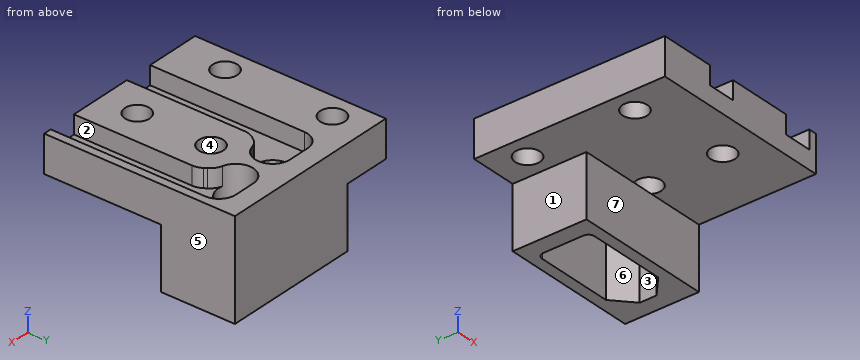
Autodesk Inventor part; units mm, degrees
ref_plane "YZ Plane" through (0, 0, 0) normal (1, 0, 0) x (0, 1, 0)
ref_plane "XZ Plane" through (0, 0, 0) normal (0, 1, 0) x (-1, 0, 0)
ref_plane "XY Plane" through (0, 0, 0) normal (0, 0, 1) x (1, 0, 0)
sketch "Эскиз1" plane through (0, 0, 0) normal (0, 0, 1) x (1, 0, 0)
  line L0 (-10, -10.5115) -> (10, -10.5115)
  line L1 (10, -10.5115) -> (10, 10.5115)
  line L2 (10, 10.5115) -> (-10, 10.5115)
  line L3 (-10, 10.5115) -> (-10, -10.5115)
  line L4 (-10, -10.5115) -> (10, 10.5115) construction
  line L5 (10, -10.5115) -> (-10, 10.5115) construction
  point P0 (0, 0)
  dimension "d0" = 20
  dimension "d1" = 21.023
extrude "Выдавливание1" add sketch "Эскиз1" along normal blind 6
sketch "Эскиз2" plane through (0, 0, 6) normal (0, 0, 1) x (1, 0, 0)
  circle A0 centre (2.5, 4.5115) radius 2.85
  circle A1 centre (-4.85, 4.5115) radius 2.85
  point P0 (0, 0)
extrude "Выдавливание2" cut sketch "Эскиз2" against normal blind 6
move faces "Перенос1" translate (-10, 0, 0) faces at (-10, 3.5038, 2)
move faces "Перенос2" translate (0, -10, 0) faces at (-10, -10.5115, 2)
sketch "Эскиз4" plane through (0, 0, 0) normal (0, 0, -1) x (-1, 0, 0)
  line L0 (8.6, 0.7615) -> (-3.85, 0.7615)
  arc A0 (8.6, 0.7615) -> (9.1, 1.2615) centre (8.6, 1.2615) ccw
  line L1 (9.1, 7.7615) -> (9.1, 1.2615)
  line L2 (-3.85, 8.2615) -> (8.6, 8.2615)
  arc A1 (9.1, 7.7615) -> (8.6, 8.2615) centre (8.6, 7.7615) ccw
  line L3 (-6.75, 5.6615) -> (-3.85, 8.2615)
  line L4 (-6.75, 3.3615) -> (-6.75, 5.6615)
  line L5 (-3.85, 0.7615) -> (-6.75, 3.3615)
  line L6 (-10, 10.5115) -> (20, 10.5115)
  line L7 (-10, 10.5115) -> (12.35, 10.5115)
  line L8 (12.35, 10.5115) -> (12.35, -1.4885)
  line L9 (12.35, -1.4885) -> (-10, -1.4885)
  line L10 (-10, -1.4885) -> (-10, 10.5115)
  point P0 (0, 0)
  dimension "d19" = 2.25
  dimension "d20" = 2.25
  dimension "d21" = 3.25
  dimension "d23" = 3.25
extrude "Выдавливание4" add sketch "Эскиз4" along normal blind 10
offset faces "Размер1" outward -0.5 faces at (-0.3, 8.2615, -3.3333) (-8.9665, 8.1016, -6.6667) (-9.1, 5.5948, -3.3333) (5.7833, 6.5282, -3.3333) (6.75, 4.1282, -3.3333) (4.8167, 1.6282, -3.3333) (-4.45, 0.7615, -3.3333) (-8.7474, 0.7837, -6.6667)
sketch "Эскиз5" plane through (0, 0, 0) normal (0, 0, -1) x (-1, 0, 0)
  circle A0 centre (16.175, 4.9639) radius 2
  line L0 (12.35, 10.5115) -> (20, 10.5115)
  point P0 (0, 0)
  point P1 (16.175, 10.5115)
  dimension "d27" = 4
extrude "Выдавливание5" cut sketch "Эскиз5" against normal blind 10
sketch "Эскиз6" plane through (0, 0, 6) normal (0, 0, 1) x (1, 0, 0)
  circle A0 centre (-16.175, -12.5115) radius 2
  circle A1 centre (-16.175, 4.9639) radius 2
  circle A2 centre (-1.1985, -0.3999) radius 2
  line L0 (-20, -20.5115) -> (10, -20.5115)
  point P0 (0, 0)
  dimension "d30" = 4
  dimension "d31" = 4
  dimension "d46" = 8
extrude "Выдавливание6" cut sketch "Эскиз6" against normal blind 6.5 contours A0
sketch "Эскиз7" plane through (0, 0, 6) normal (0, 0, 1) x (1, 0, 0)
  circle A0 centre (-4.85, 4.5115) radius 2.85
  line L0 (-4.85, 7.3615) -> (-11.0596, 7.3615)
  line L1 (-11.0596, 7.3615) -> (-11.0596, -20.5115)
  line L2 (-20, -20.5115) -> (10, -20.5115)
  line L3 (-5, 1.6655) -> (-6.4302, -0.5077)
  line L4 (-6.4302, -0.5077) -> (-6.4302, -20.5115)
  line L5 (10, 10.5115) -> (-20, 10.5115)
  line L6 (-1.175, 10.5115) -> (-1.175, 2.4545) construction
  circle A1 centre (2.5, 4.5115) radius 2.85
  line L7 (-4.85, 4.5115) -> (-4.85, 5.527) construction
  line L8 (2.5, 4.5115) -> (2.5, 5.527) construction
  line L9 (2.5, 7.3615) -> (8.7096, 7.3615)
  line L10 (8.7096, 7.3615) -> (8.7096, -20.5115)
  line L11 (2.65, 1.6655) -> (4.0802, -0.5077)
  line L12 (4.0802, -0.5077) -> (4.0802, -20.5115)
  point P0 (0, 0)
extrude "Выдавливание7" cut sketch "Эскиз7" against normal blind 3 contours A0 L3 L4 L2 L1 L0 | L12 L11 A1 L9 L10 L2
fillet "Сопряжение2" radius 2.75 6 edges at (8.7096, 7.3615, 4.5) (2.65, 1.6655, 4.5) (4.0802, -0.5077, 4.5) (-5, 1.6655, 4.5) (-6.4302, -0.5077, 4.5) (-11.0596, 7.3615, 4.5)
sketch "Эскиз8" plane through (0, 0, 6) normal (0, 0, 1) x (1, 0, 0)
  circle A0 centre (-1.175, -2.5115) radius 2
  circle A1 centre (-1.175, -14.5115) radius 2
  line L0 (-6.4302, -20.5115) -> (4.0802, -20.5115)
  circle A2 centre (-1.175, -2.5115) radius 3 construction
  point P0 (0, 0)
  point P1 (-1.175, -20.5115)
  dimension "d39" = 4
  dimension "d40" = 4
  dimension "d41" = 6
  dimension "d42" = 12
  dimension "d43" = 6
extrude "Выдавливание8" cut sketch "Эскиз8" against normal up to surface (6 mm away)
equation "\"d20\" = d19"
equation "\"d23\" = d21"
properties part number "000.012.001 - Основание"
Check sheet for the modelled part. Datum: model origin and axes. Units: mm. Face numbers are marked on the shaded views. A direction names the side the tool comes from. Round coordinates to 2 decimals unless told otherwise and drop trailing zeros. Loops run counter-clockwise (first coordinate to the right, second up) from the corner with the lowest first, then second, coordinate; pieces in that order, holes last. Notation, with made-up numbers: M -20,-27 L 33,-27 A29 ccw 33,5 Z; hole C 56,64.5 d3. An arc over 180 degrees is marked long. One line per question, with ' | ' between items. Start each with the question number.
Item 1: Gauge pin test, flat ends, axial feed: pin 1 Ø8 at (x, z) = (-5.5, -7.5) entering from -Y; pin 2 Ø2 at (x, y) = (6, -13) entering from -Z; pin 3 Ø3 at (y, z) = (5, -7) entering from -X; pin 4 Ø4.5 at (x, y) = (2.5, 4.51) entering from -Z. Record the tip position at first contact, or that the pin passes through.
Item 2: Release check for a two-part mould opening along Y. For the marked faces 5, 6 and 7 record: released by +Y, released by -Y, zero draft, split by the parting line, or undercut.
Item 3: Set-up check for the marked faces 1, 2, 3 and 4: record each of +Z, -Z, +X, -X, +Y, -Y from which the full face is reachable in a straight line by a thin tool's end or side.
Item 4: Section check B-B (y = -2). Record the boundary of the cut face in (x, z), and give its area (3 significant figures).
Item 5: Section check D-D (y = 6.5). Record the boundary of the cut face in (x, z).
Item 6: Section check A-A (z = -0.5). Record the boundary of the cut face in (x, y), and give its area (3 significant figures).
Item 7: Section check C-C (z = 3.75). State how many separate pieces and enclosed holes the cut face has, and give its area (3 significant figures).
Item 8: Scan lines: probe 1 along X at (y, z) = (-17, 4.75); probe 2 along Y at (x, z) = (-7.5, -2.75); probe 3 along X at (y, z) = (7, -3.25). Record each from-to range of solid material in increasing order.
Worked out:
1) pin 1: y = -1.49 | pin 2: z = 0 | pin 3: x = -12.35 | pin 4: through
2) face 5: zero draft | face 6: undercut | face 7: released by -Y
3) face 1: -Z, -X, +Y, -Y | face 2: +Z, -Y | face 3: -Z | face 4: +Z
4) outline: M -20,0 L -3.11,0 L -3.11,6 L -6.43,6 L -6.43,3 L -11.06,3 L -11.06,6 L -20,6 Z; M 0.76,0 L 10,0 L 10,6 L 8.71,6 L 8.71,3 L 4.08,3 L 4.08,6 L 0.76,6 Z | area: 129 mm^2
5) outline: M -20,0 L -17.46,0 L -17.46,6 L -20,6 Z; M -14.89,0 L -12.35,0 L -12.35,-10 L -9.6,-10 L -9.6,0 L -6.89,0 L -6.89,3 L -10.31,3 L -10.31,6 L -14.89,6 Z; M -2.81,0 L 0.46,0 L 0.46,6 L -2.81,6 Z; M 4.54,0 L 6.56,0 L 6.56,-10 L 10,-10 L 10,6 L 7.96,6 L 7.96,3 L 4.54,3 Z
6) outline: M -12.35,-1.49 L 10,-1.49 L 10,10.51 L -12.35,10.51 Z; hole M -9.6,1.26 A1 ccw -8.6,0.26 L 4.04,0.26 L 7.25,3.14 L 7.25,5.88 L 4.04,8.76 L -8.6,8.76 A1 ccw -9.6,7.76 Z | area: 135 mm^2
7) separate pieces: 1 | enclosed holes: 4 | area: 578 mm^2
8) probe 1: -20 to -11.06, -6.43 to 4.08, 8.71 to 10 | probe 2: -1.49 to 0.26, 8.76 to 10.51 | probe 3: -12.35 to -9.6, 6.01 to 10
